Verification items for the finished model (mm, model axes). A direction names the side the tool comes from. Give positions to 0.01 mm unless a question says otherwise; leave off trailing zeros. Loops run counter-clockwise (first coordinate to the right, second up) from the corner with the lowest first, then second, coordinate; pieces in that order, holes last. Notation, with made-up numbers: M 27.25,71 L 57.25,71 A13 ccw 57.25,77 Z; hole C 57,52 d10. An arc over 180 degrees is marked long. Use a Markdown table: item, result.
from build123d import *

# Parameters (mm, degrees)
F1_DEPTH  = 26
F2_R      = 3
F3_R      = 8
F4_DEPTH  = 23
F6_R      = 8
F7_DEPTH  = 3
F8_R      = 3
F11_DEPTH = 35


with BuildPart() as f1:
    # F0 (on Top) → F1 (new body)
    with BuildSketch(Plane.XY):
        with BuildLine():
            Line((-8, -11), (8, -11))
            ThreePointArc((8, -11), (15.0710678119, -8.0710678119), (18, -1))
            Line((18, -1), (18, 1))
            ThreePointArc((18, 1), (15.0710678119, 8.0710678119), (8, 11))
            Line((8, 11), (-8, 11))
            ThreePointArc((-8, 11), (-15.0710678119, 8.0710678119), (-18, 1))
            Line((-18, 1), (-18, -1))
            ThreePointArc((-18, -1), (-15.0710678119, -8.0710678119), (-8, -11))
        make_face()
    extrude(amount=F1_DEPTH)

    # F2
    f2_edges = [f1.edges().sort_by_distance(p)[0] for p in [
        (0, -11, 0),
        (15.071068, -8.071068, 0),
        (18, 0, 0),
        (15.071068, 8.071068, 0),
        (0, 11, 0),
        (-15.071068, 8.071068, 0),
        (-18, 0, 0),
        (-15.071068, -8.071068, 0),
    ]]
    fillet(f2_edges, radius=F2_R)

    # F3 (on face) → F4 (cut)
    with BuildSketch(Plane.XY.offset(26)):
        with Locations((8.05, 0)):
            Circle(F3_R)
        with Locations((-8.05, 0)):
            Circle(F3_R)
    extrude(amount=-F4_DEPTH, mode=Mode.SUBTRACT)

    # F6 (on offset) → F7 (join, through all)
    with BuildSketch(Plane.XY.offset(23)):
        with Locations((-8.05, 0)):
            Circle(F6_R)
        with Locations((8.05, 0)):
            Circle(F6_R)
    extrude(amount=F7_DEPTH)

    # F8
    f8_edges = [f1.edges().sort_by_distance(p)[0] for p in [
        (0, -11, 26),
        (15.071068, -8.071068, 26),
        (18, 0, 26),
        (15.071068, 8.071068, 26),
        (0, 11, 26),
        (-15.071068, 8.071068, 26),
        (-18, 0, 26),
        (-15.071068, -8.071068, 26),
    ]]
    fillet(f8_edges, radius=F8_R)

    # F10 (on offset) → F11 (cut)
    with BuildSketch(Plane.YZ.offset(19)):
        Polygon((-1, 26), (-8, 26), (-8, 24.5), (-9, 24.5), (-9, 23), (-8, 23), (8, 23), (9, 23), (9, 24.5), (8, 24.5), (8, 26), (1, 26), align=None)
    extrude(amount=-F11_DEPTH, mode=Mode.SUBTRACT)


solid = f1.part
(1) Material ranges on line 1 (Y direction, x = -8.05, z = 16.5); line 2 (X direction, y = -3.5, z = 13.5); line 3 (X direction, y = -3.25, z = 6.5), recorded low to high.
Results below:
| item | result |
|---|---|
| line 1 | -11 to -8, 8 to 11 |
| line 2 | -17.68 to -15.24, -0.86 to 0.86, 15.24 to 17.68 |
| line 3 | -17.74 to -15.36, -0.74 to 0.74, 15.36 to 17.74 |
(2) Cross-section at B-B on y = 0. Record the cut outline in (x, z).
Results below:
| item | result |
|---|---|
| outline | M -18,3 A3 ccw -15,0 L 15,0 A3 ccw 18,3 L 18,23 L 16.05,23 L 16.05,3 L 0.05,3 L 0.05,23 L -0.05,23 L -0.05,3 L -16.05,3 L -16.05,23 L -16,23 L -16,25.83 A3 ccw -18,23 Z |
(3) Cross-section at C-C on x = 3. Record the cut outline in (y, z).
Results below:
| item | result |
|---|---|
| outline | M -11,3 A3 ccw -8,0 L 8,0 A3 ccw 11,3 L 11,23 A3 ccw 8,26 L 8,24.5 L 9,24.5 L 9,23 L 6.2,23 L 6.2,3 L -6.2,3 L -6.2,23 L -9,23 L -9,24.5 L -8,24.5 L -8,26 A3 ccw -11,23 Z |
(4) Cross-section at A-A on z = 10.5. Record the cut outline in (x, y), then the cut area to 3 significant figures.
Results below:
| item | result |
|---|---|
| outline | M -18,-1 A10 ccw -8,-11 L 8,-11 A10 ccw 18,-1 L 18,1 A10 ccw 8,11 L -8,11 A10 ccw -18,1 Z; hole C -8.05,0 d16; hole C 8.05,0 d16 |
| area | 304 mm^2 |
(5) Gauge pin test, flat ends, axial feed: P1, Ø1.5, axis at y = -4, z = 21.5, coming from the +X side; P2, Ø0.8, axis at x = 3, z = 24, coming from the +Y side; P3, Ø5, axis at x = -7.5, y = 1, coming from the +Z side. Record the tip position at first contact, or that the pin passes through.
Results below:
| item | result |
|---|---|
| P1 | x = 17.74 |
| P2 | y = 10.94 |
| P3 | z = 3 |
(6) Draft check along X on faces 1 (the cylindrical face through (-15.15, -7.99, 12.86)), 2 (the flat face through (0, 0, 0)), 3 (the flat face through (8, 0, 3)). Enter one of: +X half, -X half, draft (parallel to the pull), parting line (faces both ways), or undercut.
Results below:
| item | result |
|---|---|
| face 1 | -X half |
| face 2 | draft |
| face 3 | undercut |
(7) Set-up check for faces 4 (the cylindrical face through (6.32, -7.81, 13.14)), 5 (the flat face through (0, -8, 25)), 6 (the flat face through (-16, 0, 24)): record each of +Z, -Z, +X, -X, +Y, -Y from which the full face is reachable in a straight line by a thin tool's end or side.
Results below:
| item | result |
|---|---|
| face 4 | +Z |
| face 5 | +Z, +X, -X |
| face 6 | +Z, +X, +Y, -Y |
